```python
from build123d import *

# Parameters (mm, degrees)
ESBO_O1_W                = 44.4
ESBO_O1_H                = 66
RESSALTO_EXTRUS_O1_DEPTH = 2.5
ESBO_O1_3_R              = 3
ESBO_O1_3_R_2            = 1.55
ESBO_O1_3_R_3            = 2.25
RESSALTO_EXTRUS_O2_DEPTH = 5
ESBO_O1_4_W              = 20
ESBO_O1_4_H              = 2.4
RESSALTO_EXTRUS_O3_DEPTH = 9
ESBO_O1_5_W              = 2
ESBO_O1_5_H              = 8
ESBO_O1_5_H_2            = 9.779719316
ESBO_O1_5_H_3            = 9.220608646
ESBO_O1_5_W_2            = 10.2
ESBO_O1_5_H_4            = 2.4
ESBO_O1_5_W_3            = 7
ESBO_O1_5_H_5            = 2
ESBO_O1_5_W_4            = 6.764123849
ESBO_O1_5_W_5            = 6.535876151
RESSALTO_EXTRUS_O4_DEPTH = 7
ESBO_O1_6_W              = 2
ESBO_O1_6_H              = 8
ESBO_O1_6_W_2            = 10.2
ESBO_O1_6_H_2            = 2.4
ESBO_O1_6_W_3            = 7
ESBO_O1_6_H_3            = 2
RESSALTO_EXTRUS_O5_DEPTH = 9.5


with BuildPart() as part:
    # Esboço1 → Ressalto-extrusão1 (new body)
    with BuildSketch(Plane.XY):
        with Locations((-2.493970888, -16.665150932)):
            Rectangle(ESBO_O1_W, ESBO_O1_H)
    extrude(amount=RESSALTO_EXTRUS_O1_DEPTH)

    # Esboço1<3> → Ressalto-extrusão2 (add)
    with BuildSketch(Plane.XY):
        with Locations((-15.193970888, 7.434849068)):
            Circle(ESBO_O1_3_R)
        with Locations((-15.193970888, 7.434849068)):
            Circle(ESBO_O1_3_R_2, mode=Mode.SUBTRACT)
        with Locations((10.206029112, 7.434849068)):
            Circle(ESBO_O1_3_R)
        with Locations((10.206029112, 7.434849068)):
            Circle(ESBO_O1_3_R_2, mode=Mode.SUBTRACT)
        with Locations((-19.793970888, -31.865150932)):
            Circle(ESBO_O1_3_R_3)
        with Locations((-19.793970888, -31.865150932)):
            Circle(ESBO_O1_3_R_2, mode=Mode.SUBTRACT)
        with Locations((14.806029112, -31.865150932)):
            Circle(ESBO_O1_3_R_3)
        with Locations((14.806029112, -31.865150932)):
            Circle(ESBO_O1_3_R_2, mode=Mode.SUBTRACT)
    extrude(amount=RESSALTO_EXTRUS_O2_DEPTH)

    # Esboço1<4> → Ressalto-extrusão3 (add)
    with BuildSketch(Plane.XY):
        with Locations((-2.493970888, -48.465150932)):
            Rectangle(ESBO_O1_4_W, ESBO_O1_4_H)
    extrude(amount=RESSALTO_EXTRUS_O3_DEPTH)

    # Esboço1<5> → Ressalto-extrusão4 (add)
    with BuildSketch(Plane.XY):
        Polygon((-24.693970888, 16.334849068), (-24.693970888, 6.311482938), (-22.693970888, 6.311482938), (-22.693970888, 14.334849068), (-19.793970888, 14.334849068), (-19.793970888, 16.334849068), align=None)
        with Locations((-23.693970888, 2.311482938)):
            Rectangle(ESBO_O1_5_W, ESBO_O1_5_H)
        with Locations((-23.693970888, -6.57837672)):
            Rectangle(ESBO_O1_5_W, ESBO_O1_5_H_2)
        with Locations((-23.693970888, -15.468236378)):
            Rectangle(ESBO_O1_5_W, ESBO_O1_5_H)
        with Locations((-23.693970888, -24.078540701)):
            Rectangle(ESBO_O1_5_W, ESBO_O1_5_H_3)
        with Locations((-23.693970888, -32.688845024)):
            Rectangle(ESBO_O1_5_W, ESBO_O1_5_H)
        Polygon((-24.693970888, -49.665150932), (-22.693970888, -49.665150932), (-22.693970888, -47.265150932), (-22.693970888, -36.688845024), (-24.693970888, -36.688845024), align=None)
        with Locations((-17.593970888, -48.465150932)):
            Rectangle(ESBO_O1_5_W_2, ESBO_O1_5_H_4)
        with Locations((12.606029112, -48.465150932)):
            Rectangle(ESBO_O1_5_W_2, ESBO_O1_5_H_4)
        Polygon((17.706029112, -47.265150932), (17.706029112, -49.665150932), (19.706029112, -49.665150932), (19.706029112, -36.688845024), (17.706029112, -36.688845024), align=None)
        with Locations((18.706029112, -32.688845024)):
            Rectangle(ESBO_O1_5_W, ESBO_O1_5_H)
        with Locations((18.706029112, -24.078540701)):
            Rectangle(ESBO_O1_5_W, ESBO_O1_5_H_3)
        with Locations((18.706029112, -15.468236378)):
            Rectangle(ESBO_O1_5_W, ESBO_O1_5_H)
        with Locations((18.706029112, -6.57837672)):
            Rectangle(ESBO_O1_5_W, ESBO_O1_5_H_2)
        with Locations((18.706029112, 2.311482938)):
            Rectangle(ESBO_O1_5_W, ESBO_O1_5_H)
        Polygon((17.706029112, 14.334849068), (17.706029112, 6.311482938), (19.706029112, 6.311482938), (19.706029112, 16.334849068), (14.506029112, 16.334849068), (14.506029112, 14.334849068), align=None)
        with Locations((11.006029112, 15.334849068)):
            Rectangle(ESBO_O1_5_W_3, ESBO_O1_5_H_5)
        with Locations((4.123967187, 15.334849068)):
            Rectangle(ESBO_O1_5_W_4, ESBO_O1_5_H_5)
        with Locations((-2.758094737, 15.334849068)):
            Rectangle(ESBO_O1_5_W_3, ESBO_O1_5_H_5)
        with Locations((-9.526032813, 15.334849068)):
            Rectangle(ESBO_O1_5_W_5, ESBO_O1_5_H_5)
        with Locations((-16.293970888, 15.334849068)):
            Rectangle(ESBO_O1_5_W_3, ESBO_O1_5_H_5)
    extrude(amount=RESSALTO_EXTRUS_O4_DEPTH)

    # Esboço1<6> → Ressalto-extrusão5 (add)
    with BuildSketch(Plane.XY):
        with Locations((-23.693970888, 2.311482938)):
            Rectangle(ESBO_O1_6_W, ESBO_O1_6_H)
        with Locations((-23.693970888, -15.468236378)):
            Rectangle(ESBO_O1_6_W, ESBO_O1_6_H)
        with Locations((-23.693970888, -32.688845024)):
            Rectangle(ESBO_O1_6_W, ESBO_O1_6_H)
        with Locations((-17.593970888, -48.465150932)):
            Rectangle(ESBO_O1_6_W_2, ESBO_O1_6_H_2)
        with Locations((12.606029112, -48.465150932)):
            Rectangle(ESBO_O1_6_W_2, ESBO_O1_6_H_2)
        with Locations((18.706029112, -32.688845024)):
            Rectangle(ESBO_O1_6_W, ESBO_O1_6_H)
        with Locations((18.706029112, -15.468236378)):
            Rectangle(ESBO_O1_6_W, ESBO_O1_6_H)
        with Locations((18.706029112, 2.311482938)):
            Rectangle(ESBO_O1_6_W, ESBO_O1_6_H)
        with Locations((11.006029112, 15.334849068)):
            Rectangle(ESBO_O1_6_W_3, ESBO_O1_6_H_3)
        with Locations((-2.758094737, 15.334849068)):
            Rectangle(ESBO_O1_6_W_3, ESBO_O1_6_H_3)
        with Locations((-16.293970888, 15.334849068)):
            Rectangle(ESBO_O1_6_W_3, ESBO_O1_6_H_3)
    extrude(amount=RESSALTO_EXTRUS_O5_DEPTH)


solid = part.part
```
Geometry: final body of the model. Coordinates: model frame, mm. A direction names the side the tool comes from. Round coordinates to 2 decimals unless told otherwise and drop trailing zeros. Write each loop counter-clockwise with the first axis right and the second up, starting at its lowest first coordinate (ties: lowest second). Pieces come first, ordered by that corner, then holes. Notation, with made-up numbers: M 80.25,16.25 L 112.25,16.25 A18 cw 112.25,20.25 Z; hole C 47.5,43.25 d5. An arc over 180 degrees is marked long. Answer in a Markdown table with one row per item. Add a question column.
(1) Reachability of faces 4 (the face through (18, 13, 7)), 5 (the face through (0.742, 15, 8)), 6 (the face through (-22.694, -48, 8)), 7 (the face through (-24, -24, 7)), 8 (the face through (11.5, 6.1, 5)) from +Z, -Z, +X, -X, +Y, -Y: full face, straight path, thin tool, end or side. Return the list, or none.
(2) Ray query, L1, parallel to Y at x = -5.5, z = 4; L2, parallel to X at y = -3.5, z = 3.5; L3, parallel to Z at x = -3, y = -37.5. Return the intervals inside material, ascending.
(3) Contact query for flat-ended pins moving along their axis: pin 1 (10 mm diameter, centred on x = -10.5, y = -36.5, fed in from +Z); pin 2 (0.7 mm diameter, centred on x = -5, y = -49, fed in from +Z); pin 3 (0.6 mm diameter, centred on x = 19, z = 7.5, fed in from +Y). Output: stop coordinate, or through.
(4) Cut plane A-A, the plane z = 4.25. Give the number of separate pieces and of enclosed holes in the cut face, then the cut area to 3 significant figures.
(5) Cut plane B-B, the plane y = -42. Return the cut outline in (x, z).
(6) Draft query along X for faces 1 (the face through (-19.794, 15, 8)), 2 (the face through (-3, -49.665, 5)), 3 (the face through (14.32, -34.06, 3.73)). Return one class per face: pulls with the +X half, pulls with the -X half, needs draft (parallel to the pull), parting line crosses it, or undercut.
(7) Cut plane C-C, the plane x = 5. Return the cut outline in (y, z), then the cut area to 3 significant figures.
Established:
| question | item | result |
|---|---|---|
| 1 | face 4 | +Z, +X, +Y |
| 1 | face 5 | +Z, +Y |
| 1 | face 6 | +Z, -X, -Y |
| 1 | face 7 | +Z, +X, -X |
| 1 | face 8 | +Z |
| 2 | L1 | -49.67 to -47.27, 14.33 to 16.33 |
| 2 | L2 | -24.69 to -22.69, 17.71 to 19.71 |
| 2 | L3 | 0 to 2.5 |
| 3 | pin 1 | z = 2.5 |
| 3 | pin 2 | z = 9 |
| 3 | pin 3 | y = 6.31 |
| 4 | separate pieces | 5 |
| 4 | enclosed holes | 5 |
| 4 | area | 500 mm² |
| 5 | outline | M -24.69,0 L 19.71,0 L 19.71,7 L 17.71,7 L 17.71,2.5 L -22.69,2.5 L -22.69,7 L -24.69,7 Z |
| 6 | face 1 | pulls with the -X half |
| 6 | face 2 | needs draft |
| 6 | face 3 | undercut |
| 7 | outline | M -49.67,0 L 16.33,0 L 16.33,7 L 14.33,7 L 14.33,2.5 L -47.27,2.5 L -47.27,9 L -49.67,9 Z |
| 7 | area | 190 mm² |
